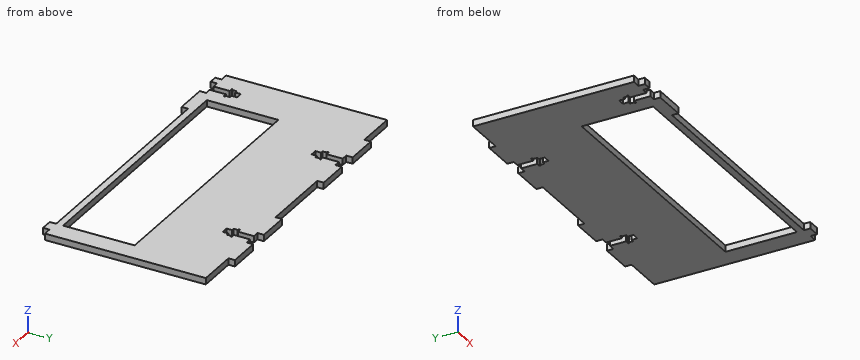
from build123d import *

# Parameters (mm, degrees)
BOSS_EXTRUDE1_DEPTH = 4
SKETCH2_W           = 158.75
SKETCH2_H           = 44.45
CUT_EXTRUDE1_DEPTH  = 6
CUT_EXTRUDE2_DEPTH  = 10
SKETCH4_W           = 5
SKETCH4_H           = 4
CUT_EXTRUDE3_DEPTH  = 10


with BuildPart() as part:
    # Sketch1 → Boss-Extrude1 (new body)
    with BuildSketch(Plane.XY):
        Polygon((-55, 50), (-43, 50), (-43, 54), (-23, 54), (-23, 50), (23, 50), (23, 54), (43, 54), (43, 50), (55, 50), (55, 54), (75, 54), (75, 50), (100, 50), (100, -50), (95, -50), (95, -54), (87.6, -54), (87.6, -50), (-58, -50), (-58, -54), (-78, -54), (-78, -50), (-90, -50), (-90, -54), (-100, -54), (-100, -50), (-100, 50), (-75, 50), (-75, 54), (-55, 54), align=None)
    extrude(amount=BOSS_EXTRUDE1_DEPTH)

    # Sketch2 → Cut-Extrude1 (cut)
    with BuildSketch(Plane(origin=(0, 0, 0), x_dir=(-1, 0, 0), z_dir=(0, 0, -1))):
        with Locations((-8.155, -23.515)):
            Rectangle(SKETCH2_W, SKETCH2_H)
    extrude(amount=-CUT_EXTRUDE1_DEPTH, mode=Mode.SUBTRACT)

    # Sketch3 → Cut-Extrude2 (cut)
    with BuildSketch(Plane(origin=(0, 0, 0), x_dir=(-1, 0, 0), z_dir=(0, 0, -1))):
        Polygon((-46.9, 50), (-51.1, 50), (-51.1, 40), (-53.5, 40), (-53.5, 39), (-52.75, 39), (-52.75, 36.5), (-51.1, 36.5), (-51.1, 33), (-46.9, 33), (-46.9, 36.5), (-45.25, 36.5), (-45.25, 39), (-44.5, 39), (-44.5, 40), (-46.9, 40), align=None)
        Polygon((51.1, 40), (51.1, 50), (46.9, 50), (46.9, 40), (44.5, 40), (44.5, 39), (45.25, 39), (45.25, 36.5), (46.9, 36.5), (46.9, 33), (51.1, 33), (51.1, 36.5), (52.75, 36.5), (52.75, 39), (53.5, 39), (53.5, 40), align=None)
        Polygon((81.9, -40), (81.9, -50), (86.1, -50), (86.1, -40), (88.5, -40), (88.5, -39), (87.75, -39), (87.75, -36.5), (86.1, -36.5), (86.1, -33), (81.9, -33), (81.9, -36.5), (80.25, -36.5), (80.25, -39), (79.5, -39), (79.5, -40), align=None)
    extrude(amount=-CUT_EXTRUDE2_DEPTH, mode=Mode.SUBTRACT)

    # Sketch4 → Cut-Extrude3 (cut)
    with BuildSketch(Plane(origin=(0, 0, 0), x_dir=(-1, 0, 0), z_dir=(0, 0, -1))):
        with Locations((97.5, -52)):
            Rectangle(SKETCH4_W, SKETCH4_H)
    extrude(amount=-CUT_EXTRUDE3_DEPTH, mode=Mode.SUBTRACT)


solid = part.part
CAD build for the part. Positions are in the model's coordinates, mm. Round coordinates to 2 decimals unless told otherwise and drop trailing zeros. Loops run counter-clockwise (first coordinate to the right, second up) from the corner with the lowest first, then second, coordinate; pieces in that order, holes last.
(1) Wall check: line 1 along X through (y, z) = (45, 2.9); line 2 along X through (y, z) = (-44, 0.6); line 3 along Y through (x, z) = (-38, 1.55). Give the ranges that are in metal, low to high.
(2) Cut at B-B (x = -5.5). Give the cut face in (y, z), plus the area to 3 significant figures.
(3) Drop flat-ended pins along their axis: pin 1 (1.9 mm diameter, centred on x = -45.5, z = 2, fed in from +Y); pin 2 (2 mm diameter, centred on y = -52, z = 2.5, fed in from +X); pin 3 (1.2 mm diameter, centred on x = -97, z = 2.5, fed in from -Y); pin 4 (10 mm diameter, centred on x = 44.5, y = -39, fed in from +Z). Give the stop position or say it passes through.
(4) Cut at A-A (y = -11.5). Give the cut face in (x, z).
Findings below:
1. line 1: x = -100 to -51.1, -46.9 to 46.9, 51.1 to 100
1. line 2: x = -100 to -86.1, -81.9 to -71.22, 87.53 to 100
1. line 3: y = -50 to -45.74, -1.29 to 54
2. outline: (-50, 0) - (-45.74, 0) - (-45.74, 4) - (-50, 4) - close; (-1.29, 0) - (50, 0) - (50, 4) - (-1.29, 4) - close
2. area: 222 mm2
3. pin 1: stops at y = 50
3. pin 2: stops at x = 95
3. pin 3: stops at y = -50
3. pin 4: passes through
4. outline: (-100, 0) - (-71.22, 0) - (-71.22, 4) - (-100, 4) - close; (87.53, 0) - (100, 0) - (100, 4) - (87.53, 4) - close
